The drawing under review shows one solid part. Ordinate dimensions are in mm from its lowest x, y, z. A direction names the side the tool comes from. Round coordinates to 2 decimals unless told otherwise and drop trailing zeros. Order: outer loops, then holes, each group sorted by start corner. A loop starts at its lowest first (then second) coordinate and runs counter-clockwise, first axis right, second up. Notation, with made-up numbers: (-14, 10.25) -> (36, 10.25) arc R10 cw to (36, 19.25) -> close; hole circle Ø3 at (36.25, 76). An arc over 180 degrees is marked (long way). Use a Markdown table: item, result. Add a question column.
1) Machinability: for the marked faces 1, 2 and 3, which of the approach directions +Z, -Z, +X, -X, +Y, -Y give a long, thin tool a straight path to every point of the face, cutting with its end or side? Answer none if there is none.
2) Draft analysis for pull direction X (two halves, no side actions). For the marked faces 4, 5, 6 and 7, state which applies: pulls with the +X half, pulls with the -X half, needs draft (parallel to the pull), parting line crosses it, or undercut.
3) Consider section C-C (y = 17.5). State the section outline as (x, z) points, plus the area to 3 significant figures.
4) Clearance check with flat-ended pins moving along their axes: P1, Ø3.5, axis at x = 7.5, z = 3.5, coming from the +Y side; P2, Ø4, axis at x = 7.5, z = 5.5, coming from the -Y side. State where each tip first meets the part, or that it passes through.
5) Wall thickness on line 1 along X through (y, z) = (1.25, 3.75); line 2 along X through (y, z) = (19, 2); line 3 along Y through (x, z) = (2.75, 4): over which ranges is each line inside the solid? List them lowest first. Write a range as [from, to].
6) Consider section D-D (x = 6.25). State the section outline as (y, z) points, plus the area to 3 significant figures.
7) Consider section A-A (y = 9.5). State the section outline as (x, z) points, plus the area to 3 significant figures.
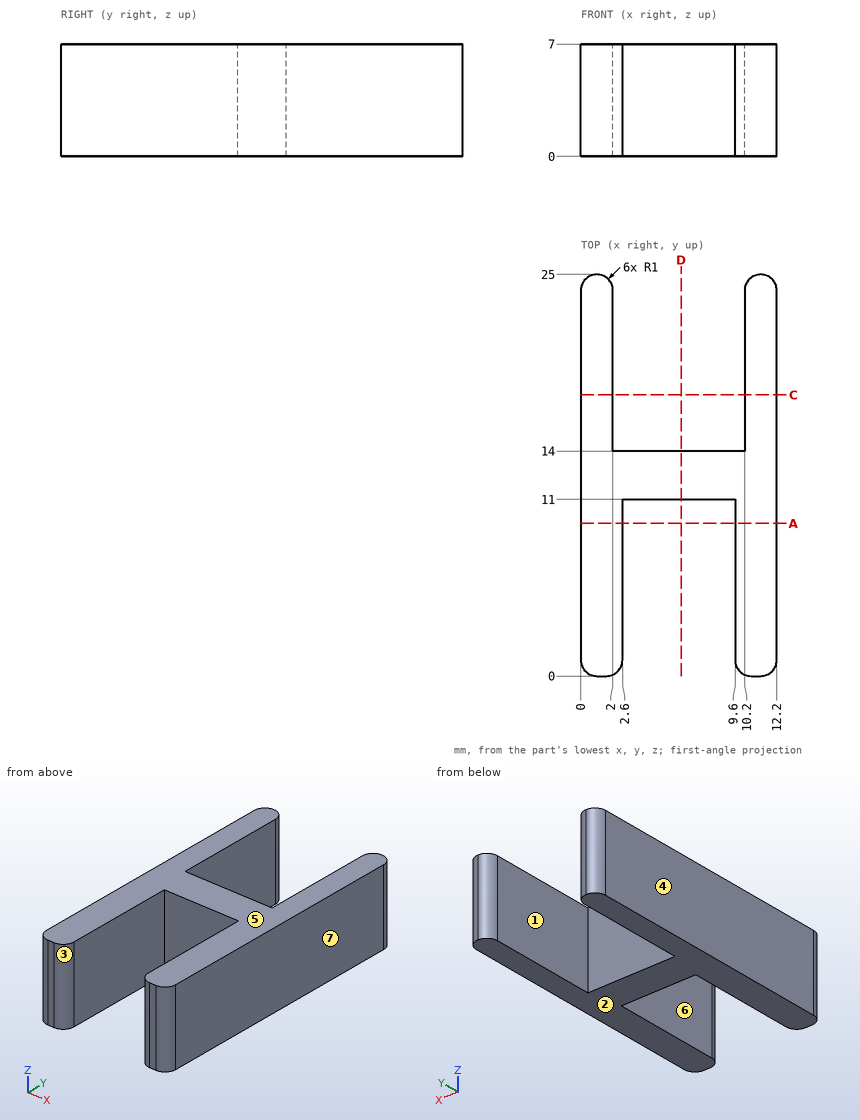
Results list:
| question | item | result |
|---|---|---|
| 1 | face 1 | +Z, -Z, +Y |
| 1 | face 2 | -Z, +X, -X, +Y, -Y |
| 1 | face 3 | +Z, -Z, -Y |
| 2 | face 4 | pulls with the -X half |
| 2 | face 5 | needs draft |
| 2 | face 6 | undercut |
| 2 | face 7 | pulls with the +X half |
| 3 | outline | (0, 0) -> (2, 0) -> (2, 7) -> (0, 7) -> close; (10.2, 0) -> (12.2, 0) -> (12.2, 7) -> (10.2, 7) -> close |
| 3 | area | 28.0 mm2 |
| 4 | P1 | y = 14 |
| 4 | P2 | y = 11 |
| 5 | line 1 | [0, 2.6], [9.6, 12.2] |
| 5 | line 2 | [0, 2], [10.2, 12.2] |
| 5 | line 3 | [11, 14] |
| 6 | outline | (11, 0) -> (14, 0) -> (14, 7) -> (11, 7) -> close |
| 6 | area | 21.0 mm2 |
| 7 | outline | (0, 0) -> (2.6, 0) -> (2.6, 7) -> (0, 7) -> close; (9.6, 0) -> (12.2, 0) -> (12.2, 7) -> (9.6, 7) -> close |
| 7 | area | 36.4 mm2 |
